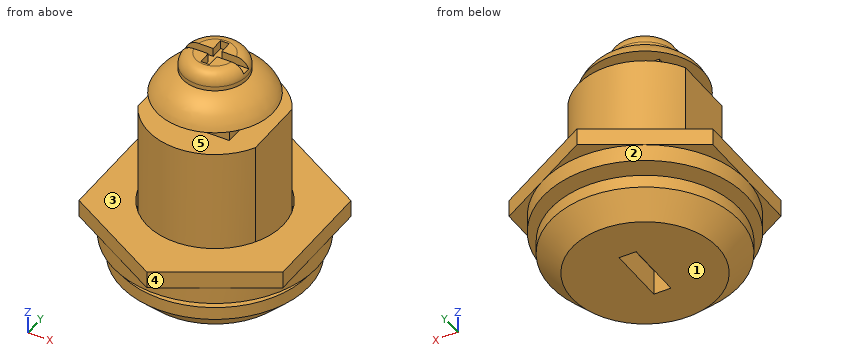
from build123d import *

# Parameters (mm, degrees)
EXTRUDE_1_DEPTH     = 17
SKETCH_3_R          = 11
EXTRUDE_2_DEPTH     = 4
CHAMFER_1_SIZE      = 2.5
SKETCH_5_W          = 8
SKETCH_5_H          = 8
EXTRUDE_4_DEPTH     = 2
SKETCH_6_R          = 2.5
EXTRUDE_5_DEPTH     = 3
SKETCH_7_R          = 3.75
EXTRUDE_6_DEPTH     = 2
FILLET_1_R          = 1.5
CUT_EXTRUDE_1_DEPTH = 1
SKETCH_9_R          = 8
EXTRUDE_7_DEPTH     = 2
SKETCH_10_W         = 2
SKETCH_10_H         = 7
CUT_EXTRUDE_2_DEPTH = 3
SKETCH_13_R         = 11.890098709
EXTRUDE_2_2_DEPTH   = 2


with BuildPart() as part:
    # 草图1 → 拉伸1 (new body)
    with BuildSketch(Plane.XY):
        with BuildLine():
            Line((6.86658576, 3.7), (6.86658576, -3.7))
            ThreePointArc((6.86658576, -3.7), (0, -7.8), (-6.86658576, -3.7))
            Line((-6.86658576, -3.7), (-6.86658576, 3.7))
            ThreePointArc((-6.86658576, 3.7), (0, 7.8), (6.86658576, 3.7))
        make_face()
    extrude(amount=EXTRUDE_1_DEPTH)

    # 草图3 → Extrude 2 (add)
    with BuildSketch(Plane(origin=(0, 0, 0), x_dir=(-1, 0, 0), z_dir=(0, 0, -1))):
        Circle(SKETCH_3_R)
    extrude(amount=EXTRUDE_2_DEPTH)

    # 倒角1
    chamfer_1_edges = [part.edges().sort_by_distance(p)[0] for p in [
        (11, 0, -4),
    ]]
    chamfer(chamfer_1_edges, length=CHAMFER_1_SIZE)

    # 草图5 → 拉伸4 (add)
    with BuildSketch(Plane.XY.offset(17)):
        Rectangle(SKETCH_5_W, SKETCH_5_H)
    extrude(amount=EXTRUDE_4_DEPTH)

    # 草图6 → 拉伸5 (add)
    with BuildSketch(Plane.XY.offset(19)):
        Circle(SKETCH_6_R)
    extrude(amount=EXTRUDE_5_DEPTH)

    # 草图7 → 拉伸6 (add)
    with BuildSketch(Plane.XY.offset(22)):
        Circle(SKETCH_7_R)
    extrude(amount=EXTRUDE_6_DEPTH)

    # 圆角1
    fillet_1_edges = [part.edges().sort_by_distance(p)[0] for p in [
        (-3.75, 0, 24),
    ]]
    fillet(fillet_1_edges, radius=FILLET_1_R)

    # 草图8 → 切除-拉伸1 (cut)
    with BuildSketch(Plane.XY.offset(24)):
        Polygon((-4.5, 0.5), (-0.5, 0.5), (-0.5, 2), (0.5, 2), (0.5, 0.5), (4.5, 0.5), (4.5, -0.5), (0.5, -0.5), (0.5, -2), (-0.5, -2), (-0.5, -0.5), (-4.5, -0.5), align=None)
    extrude(amount=-CUT_EXTRUDE_1_DEPTH, mode=Mode.SUBTRACT)

    # 草图10 → 切除-拉伸2 (cut)
    with BuildSketch(Plane(origin=(0, 0, -4), x_dir=(-1, 0, 0), z_dir=(0, 0, -1))):
        Rectangle(SKETCH_10_W, SKETCH_10_H)
    extrude(amount=-CUT_EXTRUDE_2_DEPTH, mode=Mode.SUBTRACT)

    # 草图12 → 旋转2 (revolve)
    with BuildSketch(Plane(origin=(0, 0, 0), x_dir=(0, 0, -1), z_dir=(1, 0, 0)), mode=Mode.PRIVATE) as revolve_2_sk:
        with BuildLine():
            Line((-19, 0), (-19, -6.8))
            ThreePointArc((-19, -6.8), (-21.181245185, -5.004163457), (-22, -2.3))
            Line((-22, -2.3), (-22, 0))
            Line((-22, 0), (-19, 0))
        make_face()
    revolve(revolve_2_sk.sketch.rotate(Axis((0, 0, 0), (0, 0, 1)), 270), axis=Axis((0, 0, 0), (0, 0, 1)))



with BuildPart() as body_2:
    # 草图9 → 拉伸7 (new body)
    with BuildSketch(Plane.XY.offset(3.2)):
        Polygon((11.890098709, -6.86475169), (0, -13.72950338), (-11.890098709, -6.86475169), (-11.890098709, 6.86475169), (0, 13.72950338), (11.890098709, 6.86475169), align=None)
        Circle(SKETCH_9_R, mode=Mode.SUBTRACT)
    extrude(amount=EXTRUDE_7_DEPTH)


with BuildPart() as part_1:
    add(part.part)

    add(body_2.part)  # Extrude 2 2 merges body 2
    # 草图13 → Extrude 2 2 (add)
    with BuildSketch(Plane(origin=(0, 0, 3.2), x_dir=(-1, 0, 0), z_dir=(0, 0, -1))):
        Circle(SKETCH_13_R)
    extrude(amount=EXTRUDE_2_2_DEPTH)


solid = part_1.part
Work out the finished part from the listing and answer in its coordinate system (mm). Face numbers are marked on the shaded views. A direction names the side the tool comes from. Give positions to 0.01 mm unless a question says otherwise; leave off trailing zeros. Order: outer loops, then holes, each group sorted by start corner. A loop starts at its lowest first (then second) coordinate and runs counter-clockwise, first axis right, second up. Notation, with made-up numbers: (31, -37.5) -> (39, -37.5) arc R18 cw to (39, -19.5) -> close; hole circle Ø7 at (15, -36.5). An arc over 180 degrees is marked (long way). Answer as a JSON object with one key per item and string values. Group by question number.
1. A tool of negligible diameter and unlimited length cuts with its end or side. For the marked faces 1 and 2, from which of +Z, -Z, +X, -X, +Y, -Y can it reach the whole face along a straight path? Write none if from no direction.
2. The mould has two halves that part along Z. Classify the marked faces 3, 4 and 5: released by +Z, released by -Z, zero draft, split by the parting line, or undercut.
3. Section A-A on z = 0.75 is taken. Determine the outline of the cut face in (x, y), plus the area to 3 significant figures.
4. Consider line 1 along Z through (x, y) = (-7.75, 0.5); line 2 along Y through (x, z) = (4.75, 3.5); line 3 along Z through (x, y) = (3.75, -6). Determine where each line is inside the solid, lowest interval first. Write a range as [from, to].
5. Flat-ended cylindrical pins translate along their axes: pin 1 Ø2 at (x, z) = (0, -2) entering from -Y; pin 2 Ø2 at (x, z) = (2, 6.5) entering from -Y; pin 3 Ø4 at (y, z) = (1.5, 19.5) entering from +X. Find the tip coordinate at first contact, or state that the pin passes through.
Result sheet:
{
 "1": {"face 1": "-Z, +X, -X, +Y, -Y", "face 2": "-Z"},
 "2": {"face 3": "released by +Z", "face 4": "zero draft", "face 5": "undercut"},
 "3": {"outline": "(-6.87, -3.7) arc R7.8 ccw to (6.87, -3.7) -> (6.87, 3.7) arc R7.8 ccw to (-6.87, 3.7) -> close", "area": "182 mm^2"},
 "4": {"line 1": "z = [-4, 0], [1.2, 3.2]", "line 2": "y = [-10.99, -6.44], [-6.19, 6.19], [6.44, 10.99]", "line 3": "z = [-4, 17]"},
 "5": {"pin 1": "stops at y = -11", "pin 2": "stops at y = -7.74", "pin 3": "stops at x = 6.8"}
}
